The listing builds one solid part. Answer for the finished solid, in the listing's coordinates (mm). A direction names the side the tool comes from. Give positions to 0.01 mm unless a question says otherwise; leave off trailing zeros. Loops run counter-clockwise (first coordinate to the right, second up) from the corner with the lowest first, then second, coordinate; pieces in that order, holes last.
Item 1: Consider line 1 along X through (y, z) = (-54, 0.75); line 2 along Y through (x, z) = (-0.75, 0); line 3 along Y through (x, z) = (0, 2). Determine where each line is inside the solid, lowest interval first.
Item 2: The mould has two halves that part along X. Classify faces 1 (the face through (-2.5, 29, 3)), 2 (the face through (0.1, -90.2, 0.1)), 3 (the face through (0, 31, 3)): pulls with the +X half, pulls with the -X half, needs draft (parallel to the pull), parting line crosses it, or undercut.
Item 3: A tool of negligible diameter and unlimited length cuts with its end or side. For faces 4 (the face through (-0.1, -29.8, 0.1)), 5 (the face through (0, 34.5, 0)), 6 (the face through (0, 28, 3)), 7 (the face through (-0.066, -13.885, -0.806)), 8 (the face through (2.5, 29, 3)), from which of +Z, -Z, +X, -X, +Y, -Y can it reach the whole face along a straight path? Write none if from no direction.
Item 4: Each of these flat-tipped pins is pushed along its axis until it touches: pin 1 Ø3 at (x, y) = (-2, -6.5) entering from +Z; pin 2 Ø4 at (x, z) = (-1, 3.5) entering from +Y; pin 3 Ø3.5 at (y, z) = (30, 3) entering from -X. Where does it stop, or does it pass through?
Item 5: Section C-C, the plane z = 2.75 is taken. Give the vertices of the cut face in (x, y), and give its area (3 significant figures).
Item 6: Section A-A, the plane x = 0 is taken. Give the vertices of the cut face in (y, z).
Item 7: Section B-B, the plane y = -17 is taken. Give the vertices of the cut face in (x, z).
from build123d import *

# Parameters (mm, degrees)
SKETCH1_W               = 9.4
SKETCH1_H               = 126.7
BOSS_EXTRUDE1_DEPTH     = 1
CUT_EXTRUDE2_DEPTH      = 35.5
CUT_EXTRUDE2_DEPTH_BACK = 93.2
SKETCH3_W               = 5
SKETCH3_H               = 3
BOSS_EXTRUDE2_DEPTH     = 5


with BuildPart() as part:
    # Sketch1 → Boss-Extrude1 (new body, symmetric)
    with BuildSketch(Plane.XY):
        with Locations((0, -28.85)):
            Rectangle(SKETCH1_W, SKETCH1_H)
        with BuildLine():
            ThreePointArc((-2.7, -32.5), (0, -29.8), (2.7, -32.5))
            Line((2.7, -32.5), (2.7, -87.5))
            ThreePointArc((2.7, -87.5), (0, -90.2), (-2.7, -87.5))
            Line((-2.7, -87.5), (-2.7, -32.5))
        make_face(mode=Mode.SUBTRACT)
    extrude(amount=BOSS_EXTRUDE1_DEPTH, both=True)

    # Sketch2 → Cut-Extrude2 (cut, two sides)
    with BuildSketch(Plane(origin=(0, 0, 0), x_dir=(1, 0, 0), z_dir=(0, 1, 0))) as cut_extrude2_sk:
        with BuildLine():
            ThreePointArc((-4.7, 1), (0, 0.805897581), (4.7, 1))
            Line((4.7, 1), (-4.7, 1))
        make_face()
        with BuildLine():
            Line((-4.7, 1), (4.7, 1))
            ThreePointArc((4.7, 1), (41.93387652, 19.198255851), (57, 57.805897581))
            ThreePointArc((57, 57.805897581), (-38.607641731, 99.739774101), (-4.7, 1))
        make_face()
    extrude(amount=CUT_EXTRUDE2_DEPTH, mode=Mode.SUBTRACT)
    extrude(cut_extrude2_sk.sketch, amount=-CUT_EXTRUDE2_DEPTH_BACK, mode=Mode.SUBTRACT)

    # Sketch3 → Boss-Extrude2 (add)
    with BuildSketch(Plane.XY.offset(1)):
        with Locations((0, 29.5)):
            Rectangle(SKETCH3_W, SKETCH3_H)
    extrude(amount=BOSS_EXTRUDE2_DEPTH)


solid = part.part
Worked answers:
1. line 1: x = -4.7 to -2.7, 2.7 to 4.7
1. line 2: y = -92.2 to -90.09, -29.91 to 34.5
1. line 3: y = 28 to 31
2. face 1: pulls with the -X half
2. face 2: undercut
2. face 3: needs draft
3. face 4: +Z, -Z
3. face 5: +Z, -Z, +X, -X, +Y
3. face 6: +Z, +X, -X, -Y
3. face 7: -Z, +Y, -Y
3. face 8: +Z, +X, +Y, -Y
4. pin 1: stops at z = 1
4. pin 2: stops at y = 31
4. pin 3: stops at x = -2.5
5. outline: (-2.5, 28) - (2.5, 28) - (2.5, 31) - (-2.5, 31) - close
5. area: 15.0 mm2
6. outline: (-92.2, -0.81) - (-90.2, -0.81) - (-90.2, 1) - (-92.2, 1) - close; (-29.8, -0.81) - (34.5, -0.81) - (34.5, 1) - (31, 1) - (31, 6) - (28, 6) - (28, 1) - (-29.8, 1) - close
7. outline: (-4.7, -1) arc R57 cw to (4.7, -1) - (4.7, 1) - (-4.7, 1) - close
